Design review of the part built by this model. Coordinates are the model's own, in mm. Face numbers are marked on the shaded views. Round coordinates to 2 decimals unless told otherwise and drop trailing zeros. Loops run counter-clockwise (first coordinate to the right, second up) from the corner with the lowest first, then second, coordinate; pieces in that order, holes last. Notation, with made-up numbers: (-37.75, -38.5) - (17.25, -38.5) arc R21 cw to (17.25, -11.5) - close; hole circle Ø1 at (-19, -33). An arc over 180 degrees is marked (long way). Use one line per item in the form item = value. Start each with the question number.
(1) We need section D-D, the plane x = 17.5. Write out the cut boundary in (y, z).
(2) We need section A-A, the plane z = 0. Write out the cut boundary in (x, y) (3 decimals).
(3) We need section B-B, the plane x = 30. Write out the cut boundary in (y, z) (3 decimals), then the cut area to 3 significant figures.
(4) For pin 1 (2.5 mm diameter, centred on x = -26, y = -13, fed in from -Z); pin 2 (8 mm diameter, centred on y = 6.5, z = 3, fed in from -X); pin 3 (4 mm diameter, centred on x = -18, y = -4, fed in from +Z); pin 4 (10.5 mm diameter, centred on y = -6.5, z = 9.5, fed in from +X), all flat-tipped, find the tip position at first contact; note any pin that passes through.
(5) Wall thickness on probe 1 along X at (y, z) = (0, 6); probe 2 along Y at (x, z) = (-12, 0) (3 decimals); probe 3 along Y at (x, z) = (21, 12): over which ranges is each line inside the solid? List them lowest first. Write a range as [from, to].
(6) The part is to be moulded in two halves that separate along X. For the marked faces 1, 2, 3 and 4, say which applies: released by +X, released by -X, zero draft, split by the parting line, or undercut.
(7) We need section C-C, the plane z = 7.5. Write out the cut boundary in (x, y), then the cut area to 3 significant figures.
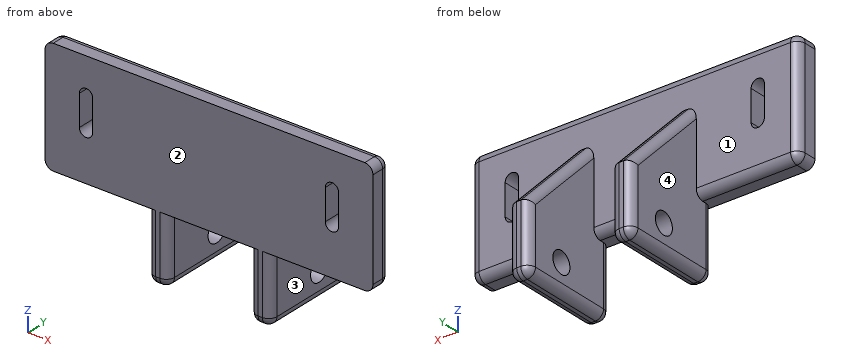
from build123d import *

# Parameters (mm, degrees)
BOSS_EXTRUDE1_START            = 10
SKETCH1_W                      = 16.5
SKETCH1_H                      = 20
SKETCH1_R                      = 2.625
BOSS_EXTRUDE1_DEPTH            = 5
BOSS_EXTRUDE2_START            = -10
SKETCH1_3_W                    = 16.5
SKETCH1_3_H                    = 20
SKETCH1_3_R                    = 2.625
BOSS_EXTRUDE2_DEPTH            = 5
BOSS_EXTRUDE3_START            = -15
SKETCH1_4_W                    = 16.5
SKETCH1_4_H                    = 5
SKETCH1_4_W_2                  = 28
BOSS_EXTRUDE3_DEPTH            = 30
SKETCH2_W                      = 25
SKETCH2_H                      = 28
BOSS_EXTRUDE4_DEPTH            = 5
CUT_EXTRUDE1_REACH             = 59.175
SKETCH1_6_W                    = 16.5
SKETCH1_6_H                    = 5
CUT_EXTRUDE1_DIRECTION_2_REACH = 59.175
BOSS_EXTRUDE5_START            = 10
BOSS_EXTRUDE5_DEPTH            = 5
BOSS_EXTRUDE6_START            = -10
BOSS_EXTRUDE6_DEPTH            = 5
FILLET1_R                      = 2


with BuildPart() as part:
    # Sketch1 → Boss-Extrude1 (new body)
    with BuildSketch(Plane(origin=(0, 0, 0), x_dir=(0, 0, -1), z_dir=(1, 0, 0)).offset(BOSS_EXTRUDE1_START)):
        with Locations((-1.75, 0)):
            Rectangle(SKETCH1_W, SKETCH1_H)
        Circle(SKETCH1_R, mode=Mode.SUBTRACT)
    extrude(amount=BOSS_EXTRUDE1_DEPTH)



with BuildPart() as body_2:
    # Sketch1<3> → Boss-Extrude2 (new body)
    with BuildSketch(Plane(origin=(0, 0, 0), x_dir=(0, 0, -1), z_dir=(1, 0, 0)).offset(BOSS_EXTRUDE2_START)):
        with Locations((-1.75, 0)):
            Rectangle(SKETCH1_3_W, SKETCH1_3_H)
        Circle(SKETCH1_3_R, mode=Mode.SUBTRACT)
    extrude(amount=-BOSS_EXTRUDE2_DEPTH)


with BuildPart() as part_1:
    add(part.part)

    add(body_2.part)  # Boss-Extrude3 merges body 2
    # Sketch1<4> → Boss-Extrude3 (add)
    with BuildSketch(Plane(origin=(0, 0, 0), x_dir=(0, 0, -1), z_dir=(1, 0, 0)).offset(BOSS_EXTRUDE3_START)):
        with Locations((-1.75, -12.5)):
            Rectangle(SKETCH1_4_W, SKETCH1_4_H)
        with Locations((-24, -12.5)):
            Rectangle(SKETCH1_4_W_2, SKETCH1_4_H)
    extrude(amount=BOSS_EXTRUDE3_DEPTH)

    # Sketch2 → Boss-Extrude4 (add)
    with BuildSketch(Plane(origin=(0, -10, 0), x_dir=(1, 0, 0), z_dir=(0, 1, 0))):
        with Locations((-27.5, -24)):
            Rectangle(SKETCH2_W, SKETCH2_H)
        with BuildLine():
            Line((-31.625, -29.25), (-31.625, -21.75))
            ThreePointArc((-31.625, -21.75), (-30, -20.125), (-28.375, -21.75))
            Line((-28.375, -21.75), (-28.375, -29.25))
            ThreePointArc((-28.375, -29.25), (-30, -30.875), (-31.625, -29.25))
        make_face(mode=Mode.SUBTRACT)
        with Locations((27.5, -24)):
            Rectangle(SKETCH2_W, SKETCH2_H)
        with BuildLine():
            Line((31.625, -29.25), (31.625, -21.75))
            ThreePointArc((31.625, -21.75), (30, -20.125), (28.375, -21.75))
            Line((28.375, -21.75), (28.375, -29.25))
            ThreePointArc((28.375, -29.25), (30, -30.875), (31.625, -29.25))
        make_face(mode=Mode.SUBTRACT)
    extrude(amount=-BOSS_EXTRUDE4_DEPTH)

    # Cut-Extrude1: up to this face of the body (flat: up to its plane)
    cut_extrude1_end = Plane(part_1.part.faces().sort_by_distance((10, 0, -6.240722157))[0])
    # Sketch1<6> → Cut-Extrude1 (cut, up to the picked face)
    with BuildSketch(Plane(origin=(0, 0, 0), x_dir=(0, 0, -1), z_dir=(1, 0, 0)), mode=Mode.PRIVATE) as cut_extrude1_sk1:
        with Locations((-1.75, -12.5)):
            Rectangle(SKETCH1_6_W, SKETCH1_6_H)
    cut_extrude1_tool1 = split(extrude(cut_extrude1_sk1.sketch, amount=CUT_EXTRUDE1_REACH, mode=Mode.PRIVATE), bisect_by=cut_extrude1_end, keep=Keep.BOTH, mode=Mode.PRIVATE)
    add(cut_extrude1_tool1.solids().sort_by(Axis((0, -12.5, 1.75), (1, 0, 0)))[0], mode=Mode.SUBTRACT)

    # Cut-Extrude1 direction 2: up to this face of the body (flat: up to its plane)
    cut_extrude1_direction_2_end = Plane(part_1.part.faces().sort_by_distance((-10, 0, -6.240722157))[0])
    # Sketch1<6> → Cut-Extrude1 direction 2 (cut, up to the picked face)
    with BuildSketch(Plane(origin=(0, 0, 0), x_dir=(0, 0, -1), z_dir=(1, 0, 0)), mode=Mode.PRIVATE) as cut_extrude1_direction_2_sk1:
        with Locations((-1.75, -12.5)):
            Rectangle(SKETCH1_6_W, SKETCH1_6_H)
    cut_extrude1_direction_2_tool1 = split(extrude(cut_extrude1_direction_2_sk1.sketch, amount=-CUT_EXTRUDE1_DIRECTION_2_REACH, mode=Mode.PRIVATE), bisect_by=cut_extrude1_direction_2_end, keep=Keep.BOTH, mode=Mode.PRIVATE)
    add(cut_extrude1_direction_2_tool1.solids().sort_by(Axis((0, -12.5, 1.75), (-1, 0, 0)))[0], mode=Mode.SUBTRACT)

    # Sketch1<7> → Boss-Extrude5 (add)
    with BuildSketch(Plane(origin=(0, 0, 0), x_dir=(0, 0, -1), z_dir=(1, 0, 0)).offset(BOSS_EXTRUDE5_START)):
        Polygon((-30, -10), (-10, -10), (-10, 10), align=None)
    extrude(amount=BOSS_EXTRUDE5_DEPTH)

    # Sketch1<8> → Boss-Extrude6 (add)
    with BuildSketch(Plane(origin=(0, 0, 0), x_dir=(0, 0, -1), z_dir=(1, 0, 0)).offset(BOSS_EXTRUDE6_START)):
        Polygon((-30, -10), (-10, -10), (-10, 10), align=None)
    extrude(amount=-BOSS_EXTRUDE6_DEPTH)

    # Fillet1
    fillet1_edges = [part_1.edges().sort_by_distance(p)[0] for p in [
        (12.5, 10, -6.5),
        (-10, 0, 20),
        (-15, 0, 20),
        (12.5, -15, -6.5),
        (-15, -2.5, -6.5),
        (0, -10, 38),
        (-15, -15, 1.75),
        (15, -2.5, -6.5),
        (15, 10, 1.75),
        (-10, 10, 1.75),
        (-10, -2.5, -6.5),
        (-12.5, 10, -6.5),
        (-15, 10, 1.75),
        (15, -15, 1.75),
        (-40, -12.5, 38),
        (-40, -12.5, 10),
        (-40, -10, 24),
        (-27.5, -10, 10),
        (27.5, -10, 10),
        (40, -12.5, 10),
        (40, -10, 24),
        (40, -12.5, 38),
        (10, 10, 1.75),
        (10, -2.5, -6.5),
        (-12.5, -15, -6.5),
        (10, -15, 1.75),
        (0, -10, 10),
        (-10, -15, 1.75),
        (10, 0, 20),
        (15, 0, 20),
    ]]
    fillet(fillet1_edges, radius=FILLET1_R)


solid = part_1.part
Data:
q1.outline = (-15, 10) - (-12, 10) arc R2 ccw to (-10, 12) - (-10, 36) arc R2 ccw to (-12, 38) - (-15, 38) - close
q2.outline = (-15, -13) arc R2 ccw to (-13, -15) - (-12, -15) arc R2 ccw to (-10, -13) - (-10, -2.625) - (-15, -2.625) - close; (-15, 2.625) - (-10, 2.625) - (-10, 8) arc R2 ccw to (-12, 10) - (-13, 10) arc R2 ccw to (-15, 8) - close; (10, -13) arc R2 ccw to (12, -15) - (13, -15) arc R2 ccw to (15, -13) - (15, -2.625) - (10, -2.625) - close; (10, 2.625) - (15, 2.625) - (15, 8) arc R2 ccw to (13, 10) - (12, 10) arc R2 ccw to (10, 8) - close
q3.outline = (-15, 10) - (-12, 10) arc R2 ccw to (-10, 12) - (-10, 20.125) - (-15, 20.125) - close; (-15, 30.875) - (-10, 30.875) - (-10, 36) arc R2 ccw to (-12, 38) - (-15, 38) - close
q3.area = 84.5 mm^2
q4.pin_1 = 10
q4.pin_2 = -15
q4.pin_3 = through
q4.pin_4 = 39.84
q5.probe_1 = [-15, -10], [10, 15]
q5.probe_2 = [-15, -2.625], [2.625, 10]
q5.probe_3 = [-15, -10]
q6.face_1 = undercut
q6.face_2 = zero draft
q6.face_3 = released by +X
q6.face_4 = released by -X
q7.outline = (-15, -13) arc R2 ccw to (-13, -15) - (-12, -15) arc R2 ccw to (-10, -13) - (-10, 8) arc R2 ccw to (-12, 10) - (-13, 10) arc R2 ccw to (-15, 8) - close; (10, -13) arc R2 ccw to (12, -15) - (13, -15) arc R2 ccw to (15, -13) - (15, 8) arc R2 ccw to (13, 10) - (12, 10) arc R2 ccw to (10, 8) - close
q7.area = 243 mm^2
